from build123d import *

# Parameters (mm, degrees)
BOSS_EXTRUDE1_DEPTH  = 150
SKETCH3_W            = 943.281144354
SKETCH3_H            = 2008.356165054
BOSS_EXTRUDE2_DEPTH  = 125
SKETCH4_W            = 877.751971552
SKETCH4_H            = 195.909630412
BOSS_EXTRUDE3_DEPTH  = 670
CUT_EXTRUDE1_DEPTH   = 1095
SKETCH6_R            = 20.377587803
BOSS_EXTRUDE4_DEPTH  = 40
SKETCH7_W            = 40.755175605
SKETCH7_H            = 40.755175605
CUT_EXTRUDE2_DEPTH   = 10
LPATTERN1_COUNT      = 2
LPATTERN1_PITCH      = 670
LPATTERN1_COUNT_DIR2 = 2
LPATTERN1_PITCH_DIR2 = 1065
SKETCH9_W            = 206.090065038
SKETCH9_H            = 55.535964875
CUT_EXTRUDE3_DEPTH   = 40
SKETCH10_W           = 145.11063413
SKETCH10_H           = 10
CUT_EXTRUDE4_DEPTH   = 40


with BuildPart() as part:
    # Sketch1 → Boss-Extrude1 (new body)
    with BuildSketch(Plane(origin=(0, 0, 0), x_dir=(1, 0, 0), z_dir=(0, 1, 0))):
        with BuildLine():
            Line((-535, 910), (-535, -910))
            ThreePointArc((-535, -910), (-488.13708499, -1023.13708499), (-375, -1070))
            Line((-375, -1070), (375, -1070))
            ThreePointArc((375, -1070), (488.13708499, -1023.13708499), (535, -910))
            Line((535, -910), (535, 910))
            ThreePointArc((535, 910), (488.13708499, 1023.13708499), (375, 1070))
            Line((375, 1070), (-375, 1070))
            ThreePointArc((-375, 1070), (-488.13708499, 1023.13708499), (-535, 910))
        make_face()
        with BuildLine():
            Line((-375, 990), (375, 990))
            ThreePointArc((375, 990), (431.568542495, 966.568542495), (455, 910))
            Line((455, 910), (455, -910))
            ThreePointArc((455, -910), (431.568542495, -966.568542495), (375, -990))
            Line((375, -990), (-375, -990))
            ThreePointArc((-375, -990), (-431.568542495, -966.568542495), (-455, -910))
            Line((-455, -910), (-455, 910))
            ThreePointArc((-455, 910), (-431.568542495, 966.568542495), (-375, 990))
        make_face(mode=Mode.SUBTRACT)
    extrude(amount=BOSS_EXTRUDE1_DEPTH)

    # Sketch3 → Boss-Extrude2 (add)
    with BuildSketch(Plane.XZ):
        Rectangle(SKETCH3_W, SKETCH3_H)
    extrude(amount=-BOSS_EXTRUDE2_DEPTH)

    # Sketch4 → Boss-Extrude3 (add)
    with BuildSketch(Plane.XZ):
        with Locations((0, 533.469606343)):
            Rectangle(SKETCH4_W, SKETCH4_H)
        with Locations((0, -533.469606343)):
            Rectangle(SKETCH4_W, SKETCH4_H)
    extrude(amount=BOSS_EXTRUDE3_DEPTH)

    # Sketch5 → Cut-Extrude1 (cut)
    with BuildSketch(Plane(origin=(438.875985776, 0, 0), x_dir=(0, 0, -1), z_dir=(1, 0, 0))):
        Polygon((-576.492082972, -597.71526573), (-631.424421549, 0), (-813.99135503, -798.682277913), (-322.424833628, -798.682277913), (-435.514791137, 0), (-489.780888803, -597.71526573), align=None)
        Polygon((435.514791137, 0), (489.780888803, -597.71526573), (576.492082972, -597.71526573), (631.424421549, 0), (813.99135503, -798.682277913), (322.424833628, -798.682277913), align=None)
    extrude(amount=-CUT_EXTRUDE1_DEPTH, mode=Mode.SUBTRACT)

    # Sketch6 → Boss-Extrude4 (add)
    with BuildSketch(Plane.XZ.offset(597.71526573)):
        with Locations((334.358840028, -533.469606343)):
            Circle(SKETCH6_R)
        with Locations((-334.358840028, -533.469606343)):
            Circle(SKETCH6_R)
        with Locations((-334.358840028, 533.469606343)):
            Circle(SKETCH6_R)
        with Locations((334.358840028, 533.469606343)):
            Circle(SKETCH6_R)
    extrude(amount=BOSS_EXTRUDE4_DEPTH)

    # Sketch7 → Cut-Extrude2 (cut)
    with BuildSketch(Plane.XZ.offset(637.71526573)):
        with Locations((354.736427831, -533.469606343)):
            Rectangle(SKETCH7_W, SKETCH7_H)
    extrude(amount=-CUT_EXTRUDE2_DEPTH, mode=Mode.SUBTRACT)

    # Sketch8 → Revolve1 (revolve)
    with BuildSketch(Plane(origin=(334.358840028, 0, 0), x_dir=(0, 0, -1), z_dir=(1, 0, 0))):
        Polygon((513.09201854, -627.71526573), (511.526412773, -633.680135283), (507.420377104, -640.04449057), (500.234814684, -643.226668213), (490.175027295, -644.86908248), (483.194766658, -644.86908248), (483.194766658, -651.028135984), (533.469606343, -651.028135984), (533.469606343, -627.71526573), align=None)
    revolve1 = revolve(axis=Axis((334.358840028, -651.028135984, -533.469606343), (0, 1, 0)))

    # LPattern1: Revolve1 2 × 2
    with Locations(*[(-i * LPATTERN1_PITCH, 0, j * LPATTERN1_PITCH_DIR2) for i in range(LPATTERN1_COUNT) for j in range(LPATTERN1_COUNT_DIR2) if (i, j) != (0, 0)]):
        add(revolve1)

    # Sketch9 → Cut-Extrude3 (cut)
    with BuildSketch(Plane.XY.offset(1070)):
        with Locations((0, 62.871676898)):
            Rectangle(SKETCH9_W, SKETCH9_H)
    cut_extrude3 = extrude(amount=-CUT_EXTRUDE3_DEPTH, mode=Mode.SUBTRACT)

    # Sketch10 → Cut-Extrude4 (cut)
    with BuildSketch(Plane(origin=(0, 0, 990), x_dir=(-1, 0, 0), z_dir=(0, 0, -1))):
        with Locations((0, 129.886472927)):
            Rectangle(SKETCH10_W, SKETCH10_H)
    cut_extrude4 = extrude(amount=-CUT_EXTRUDE4_DEPTH, mode=Mode.SUBTRACT)

    # Mirror1: Cut-Extrude3, Cut-Extrude4 across plane
    add(cut_extrude3.mirror(Plane.XY), mode=Mode.SUBTRACT)
    add(cut_extrude4.mirror(Plane.XY), mode=Mode.SUBTRACT)


solid = part.part
Here's how the part is built. I have some questions about the finished solid (model axes, mm). A direction names the side the tool comes from. Coordinates: 2 decimals unless noted, no trailing zeros. Write each loop counter-clockwise with the first axis right and the second up, starting at its lowest first coordinate (ties: lowest second). Pieces come first, ordered by that corner, then holes. Notation, with made-up numbers: (-6.75, -24.5) - (16.25, -24.5) arc R15 cw to (16.25, -0.5) - close; hole circle Ø11 at (21, 49.5). An arc over 180 degrees is marked (long way). Use one line per item in the form item = value.
1) On a 3-axis mill with a long thin cutter (end or side, diameter ignored), from which of +Z, -Z, +X, -X, +Y, -Y can I reach the whole of each face in a straight line? I mean faces 4 (the flat face through (-1, 35.104, -1050)), 5 (the flat face through (438.876, -228, -535)), 6 (the cylindrical face through (-430.94, 137.32, 967.19)), 7 (the flat face through (-294, -644.869, 517)), 8 (the cylindrical face through (-333.431, -647.992, 481.304)). Say none if no direction works.
Solved:
face_4 = -Z
face_5 = +Z, -Z, +X, -Y
face_6 = +Y
face_7 = none
face_8 = -Y
2) Thinking about a two-plate mould opening in X: for faces 1 (the cylindrical face through (-486.89, 73.95, -1024.37)), 2 (the flat face through (6.144, -303.042, -603.574)), 3 (the flat face through (-103.045, 62, 1050)), which applies, released by +X, released by -X, zero draft, split by the parting line, or undercut?
Solved:
face_1 = released by -X
face_2 = zero draft
face_3 = undercut
3) Suppose I cut it at D-D, the plane y = 61. Write out the boundary of the cut face in (x, z).
Solved:
outline = (-535, -910) arc R160 ccw to (-375, -1070) - (-103.05, -1070) - (-103.05, -1030) - (103.05, -1030) - (103.05, -1070) - (375, -1070) arc R160 ccw to (535, -910) - (535, 910) arc R160 ccw to (375, 1070) - (103.05, 1070) - (103.05, 1030) - (-103.05, 1030) - (-103.05, 1070) - (-375, 1070) arc R160 ccw to (-535, 910) - close
4) Suppose I cut it at B-B, the plane x = 163. Write out the boundary of the cut face in (y, z).
Solved:
outline = (-597.72, -576.49) - (0, -631.42) - (0, -1070) - (150, -1070) - (150, -990) - (125, -990) - (125, 990) - (150, 990) - (150, 1070) - (0, 1070) - (0, 631.42) - (-597.72, 576.49) - (-597.72, 489.78) - (0, 435.51) - (0, -435.51) - (-597.72, -489.78) - close
5) Suppose I cut it at C-C, the plane z = -8.5. Write out the boundary of the cut face in (x, y).
Solved:
outline = (-535, 0) - (535, 0) - (535, 150) - (455, 150) - (455, 125) - (-455, 125) - (-455, 150) - (-535, 150) - close
6) I need wall thicknesses on line 1 (Y direction, x = -141, z = 558.5); line 2 (Y direction, x = -220.5, z = -748.5); line 3 (Z direction, x = 301, y = -312). Which ranges of each line are inside material? Lowest first, please.
Solved:
line_1 = -597.72 to 125
line_2 = 0 to 125
line_3 = -602.75 to -463.84, 463.84 to 602.75
7) I'm going to push flat-ended pins straight in: P1, Ø6, axis at x = 120, z = 160.5, coming from the +Y side; P2, Ø3, axis at x = 99, z = 789.5, coming from the -Y side; P3, Ø5, axis at x = 385.5, y = 19, coming from the -Z side. Where does each tip first touch, or does it pass through?
Solved:
P1 = 125
P2 = 0
P3 = -1069.8
8) Suppose I cut it at A-A, the plane y = -510.5. Write out the boundary of the cut face in (x, z), plus the area to 3 significant figures.
Solved:
outline = (-438.88, -584.51) - (438.88, -584.51) - (438.88, -481.86) - (-438.88, -481.86) - close; (-438.88, 481.86) - (438.88, 481.86) - (438.88, 584.51) - (-438.88, 584.51) - close
area = 180,000 mm2
